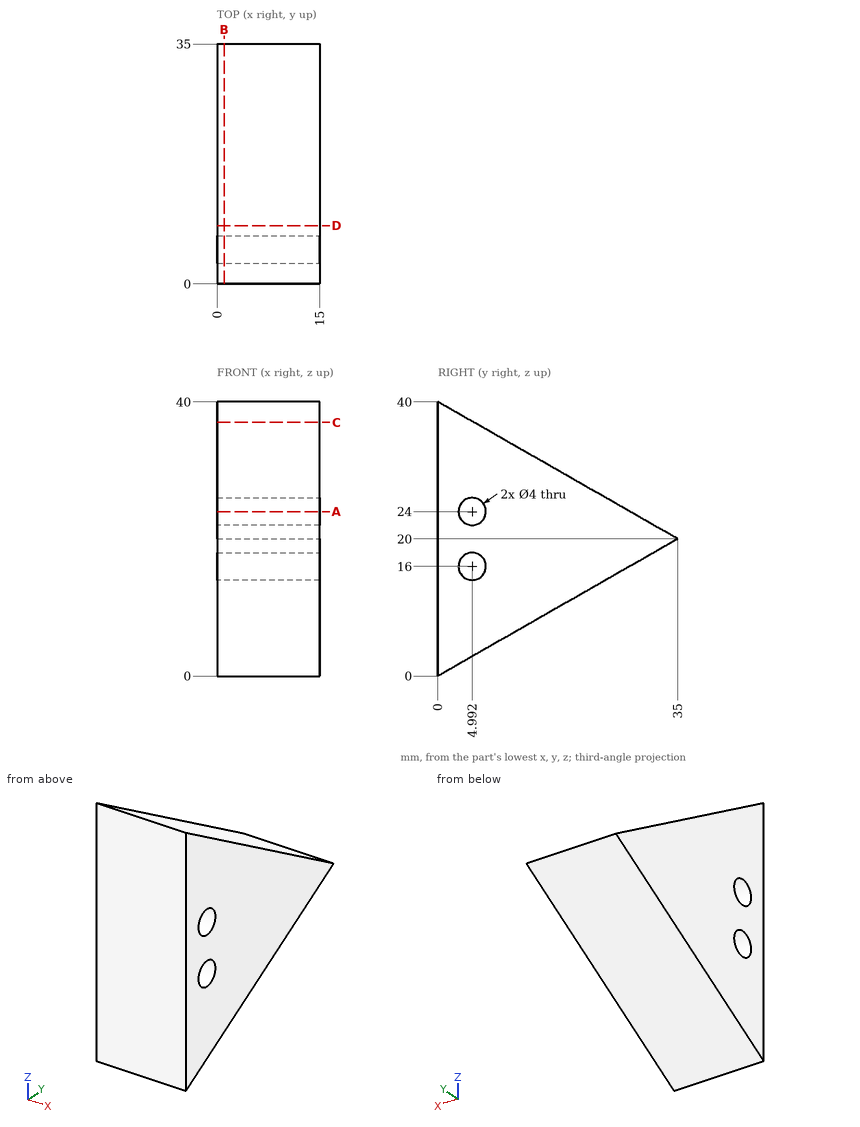
Print and shaded views of the part. All mm, measured from the part's lowest x, y and z. Coordinates: 2 decimals unless noted, no trailing zeros. Order: outer loops, then holes, each group sorted by start corner. A loop starts at its lowest first (then second) coordinate and runs counter-clockwise, first axis right, second up. Notation, with made-up numbers: (75, 65) - (88, 65) arc R18 ccw to (88, 76) - close; hole circle Ø7 at (41, -34). An arc over 180 degrees is marked (long way). Put each result on its own line as item: value.
1. Probe line 1 along Y through (x, z) = (6.5, 16); line 2 along Y through (x, z) = (4.75, 37); line 3 along Z through (x, y) = (10.25, 23). List the from-to ranges inside material, lowest first. Write a range as [from, to].
Answer sheet:
line 1: y = [0, 2.99], [6.99, 28]
line 2: y = [0, 5.25]
line 3: z = [13.14, 26.86]
2. Saw through at D-D (y = 8.5). Write the cut outline in (x, z).
Answer sheet:
outline: (0, 4.86) - (15, 4.86) - (15, 35.14) - (0, 35.14) - close
3. Drop flat-ended pins along their axis: P1, Ø1, axis at x = 12.5, y = 10.5, coming from the -Z side; P2, Ø3, axis at y = 4.99, z = 16, coming from the +X side; P3, Ø8, axis at x = 12, z = 13.5, coming from the +Y side (1 decimal); P4, Ø1.5, axis at x = 3, z = 34.5, coming from the +Y side. Give the stop position or say it passes through.
Answer sheet:
P1: stops at z = 5.71
P2: passes through
P3: stops at y = 30.6
P4: stops at y = 10.94
4. Saw through at C-C (z = 37). Write the cut outline in (x, y).
Answer sheet:
outline: (0, 0) - (15, 0) - (15, 5.25) - (0, 5.25) - close
5. Saw through at A-A (z = 24). Write the cut outline in (x, y).
Answer sheet:
outline: (0, 0) - (15, 0) - (15, 2.99) - (0, 2.99) - close; (0, 6.99) - (15, 6.99) - (15, 28) - (0, 28) - close
6. Saw through at B-B (x = 1). Write the cut outline in (y, z), and give its area (3 significant figures).
Answer sheet:
outline: (0, 0) - (35, 20) - (0, 40) - close; hole circle Ø4 at (4.99, 16); hole circle Ø4 at (4.99, 24)
area: 675 mm^2
